Read the model definition and answer for the solid it produces. Units are mm, in the model's axes. Coordinates: 2 decimals unless noted, no trailing zeros. Order: outer loops, then holes, each group sorted by start corner. A loop starts at its lowest first (then second) coordinate and runs counter-clockwise, first axis right, second up. Notation, with made-up numbers: M -25,65.5 L 32,65.5 A21 ccw 32,70.5 Z; hole C 46,27 d8. An arc over 180 degrees is marked long. Use a Markdown table: item, result. Add a question column.
1) Find section B-B on z = -1.25. Write down the section's boundary in (x, y).
2) The mould has two halves that part along X. Classify faces 1 (the face through (0, 0, -9)), 2 (the face through (0, 2, -8)), 3 (the face through (-13.51, 2, -6)): released by +X, released by -X, zero draft, split by the parting line, or undercut.
3) Find section C-C on x = 10.97. Write down the section's boundary in (y, z).
4) Find the intervals of material crossed by probe 1 along Y at (x, z) = (10.97, -6); probe 2 along X at (y, z) = (1.5, -2.25); probe 3 along X at (y, z) = (3.65, -4), in increasing order. Write a range as [from, to].
Autodesk Fusion 360 part; units mm, degrees
sketch "Sketch1" plane through (0, 0, 0) normal (0, 1, 0) x (1, 0, 0)
  circle A0 centre (0, 0) radius 8
  line L0 (-7.9964, 0.24) -> (-13.51, 0.24)
  line L1 (-13.51, 0.24) -> (-13.51, 11)
  line L2 (-13.51, 11) -> (13.51, 11)
  line L3 (13.51, 11) -> (13.51, 0.24)
  line L4 (13.51, 0.24) -> (7.9964, 0.24)
  point P0 (0, 8)
  dimension "d1" = 27.02
  dimension "d2" = 10.76
  dimension "d3" = 16
  dimension "d4" = 3
extrude "Extrude1" add sketch "Sketch1" along normal blind 5 contours A0 L0 L1 L2 L3 L4
sketch "Sketch2" plane through (0, 0, -11) normal (0, 0, -1) x (1, 0, 0)
  line L0 (13.51, 0) -> (-13.51, 0)
  line L1 (-13.51, 0) -> (-13.51, -5)
  line L2 (-13.51, -5) -> (13.51, -5)
  line L3 (13.51, -5) -> (13.51, 0)
  line L4 (-10.97, -2.5) -> (10.97, -2.5) construction
  point P0 (13.51, -2.5)
  point P1 (0, -2.5)
  dimension "d7" = 21.94
hole "Hole1" at (-10.97, 2.5, -11) at (10.97, 2.5, -11) direction (0, 0, 1) diameter 2.9 end through all
Check result:
| question | item | result |
|---|---|---|
| 1 | outline | M -13.51,0 L -7.9,0 L -7.9,5 L -13.51,5 Z; M 7.9,0 L 13.51,0 L 13.51,5 L 7.9,5 Z; hole C -10.97,2.5 d2.9; hole C 10.97,2.5 d2.9 |
| 2 | face 1 | zero draft |
| 2 | face 2 | undercut |
| 2 | face 3 | released by -X |
| 3 | outline | M 0,-11 L 1.05,-11 L 1.05,-0.24 L 0,-0.24 Z; M 3.95,-11 L 5,-11 L 5,-0.24 L 3.95,-0.24 Z |
| 4 | probe 1 | y = [0, 1.05], [3.95, 5] |
| 4 | probe 2 | x = [-13.51, -12.02], [-9.92, -7.68], [7.68, 9.92], [12.02, 13.51] |
| 4 | probe 3 | x = [-13.51, -11.85], [-10.09, -6.93], [6.93, 10.09], [11.85, 13.51] |
